```python
from build123d import *

# Parameters (mm, degrees)
SKETCH2_W                = 21
SKETCH2_H                = 21
BOSS_EXTRUDE1_DEPTH      = 300
BOSS_EXTRUDE1_DEPTH_BACK = 100
SKETCH3_W                = 16
SKETCH3_H                = 16
CUT_EXTRUDE1_DEPTH       = 800
SKETCH14_R               = 2.5
BOSS_EXTRUDE3_DEPTH      = 10
LPATTERN1_COUNT          = 3
LPATTERN1_PITCH          = 120


with BuildPart() as part:
    # Sketch2 → Boss-Extrude1 (new body, two sides)
    with BuildSketch(Plane(origin=(0, 0, 0), x_dir=(1, 0, 0), z_dir=(0, 1, 0))) as boss_extrude1_sk:
        Rectangle(SKETCH2_W, SKETCH2_H)
    extrude(amount=BOSS_EXTRUDE1_DEPTH)
    extrude(boss_extrude1_sk.sketch, amount=-BOSS_EXTRUDE1_DEPTH_BACK)

    # Sketch3 → Cut-Extrude1 (cut)
    with BuildSketch(Plane.XZ.offset(100)):
        Rectangle(SKETCH3_W, SKETCH3_H)
    extrude(amount=-CUT_EXTRUDE1_DEPTH, mode=Mode.SUBTRACT)

    # Sketch14 → Boss-Extrude3 (add)
    with BuildSketch(Plane(origin=(9.15884387, 19.641204062, 19.641204062), x_dir=(0.949705125, -0.221427386, -0.221427386), z_dir=(0.313145613, 0.671542934, 0.671542934))):
        Polygon((-12.902384486, 16.967939861), (98.008310235, -50.846644091), (103.224816692, -42.31505219), (-7.685878028, 25.499531762), align=None)
        with Locations((87.819175611, -38.756088454)):
            Circle(SKETCH14_R, mode=Mode.SUBTRACT)
    boss_extrude3 = extrude(amount=-BOSS_EXTRUDE3_DEPTH)

    # LPattern1: Boss-Extrude3 ×3
    with Locations(*[(0, i * LPATTERN1_PITCH, 0) for i in range(1, LPATTERN1_COUNT)]):
        add(boss_extrude3)


solid = part.part
```
The listing builds one solid part. Answer for the finished solid, in the listing's coordinates (mm). A direction names the side the tool comes from. Round coordinates to 2 decimals unless told otherwise and drop trailing zeros. Loops run counter-clockwise (first coordinate to the right, second up) from the corner with the lowest first, then second, coordinate; pieces in that order, holes last. Notation, with made-up numbers: (74, -30) - (78, -30) arc R27 cw to (78, -10) - close; hole circle Ø3 at (25, 35). An arc over 180 degrees is marked (long way). Use one line per item in the form item = value. Start each with the question number.
1. For a pull along X with two mould halves and no side action, classify faces 1 (the face through (-10.5, 103, 0)), 2 (the face through (103.136, -38.921, 27.039)), 3 (the face through (0, 103, -10.5)), 4 (the face through (0, 97, 8)) as pulls with the +X half, pulls with the -X half, needs draft (parallel to the pull), parting line crosses it, or undercut.
2. A tool of negligible diameter and unlimited length cuts with its end or side. For faces 5 (the face through (-2.127, 273.659, 3.545)), 6 (the face through (51.8, -1.1, 20.5)), 7 (the face through (53.6, 232.11, 11.56)), 8 (the face through (4, 153.5, 0.8)), 9 (the face through (57.98, 116.37, 12.81)), from which of +Z, -Z, +X, -X, +Y, -Y can it reach the whole face along a straight path? Write none if from no direction.
3. The part is cut by section B-B on y = 226.5. Determine the outline of the cut face in (x, z).
4. The part is cut by section A-A on y = -68.5. Determine the outline of the cut face in (x, z).
5. Given pin 1 Ø6 at (y, z) = (255.5, 20.5) entering from -X; pin 2 Ø10.5 at (y, z) = (57, -2) entering from +X; pin 3 Ø1.5 at (x, y) = (29.5, 127.5) entering from -Z; pin 4 Ø17.5 at (x, y) = (1, 75.5) entering from +Z, each flat-ended and moving along its own axis, determine where each tip first touches the part or whether it passes through.
6. The part is cut by section C-C on x = 20. Determine the outline of the cut face in (y, z).
7. Consider line 1 (X direction, y = 262, z = -1.5); line 2 (Y direction, x = 36, z = 14.5); line 3 (Y direction, x = 5.5, z = 12). Determine where each line is inside the solid, lowest interval first. Write a range as [from, to].
Geometry check:
q1.face_1 = pulls with the -X half
q1.face_2 = pulls with the +X half
q1.face_3 = needs draft
q1.face_4 = undercut
q2.face_5 = +Y
q2.face_6 = +Z, +X
q2.face_7 = -Z
q2.face_8 = none
q2.face_9 = -Z, +X
q3.outline = (-10.5, -10.5) - (10.5, -10.5) - (10.5, 10.5) - (-10.5, 10.5) - close; (53.74, 17.1) - (65.78, 11.49) - (78.67, 20.37) - (66.63, 25.98) - close; hole (-8, -8) - (8, -8) - (8, 8) - (-8, 8) - close
q4.outline = (-10.5, -10.5) - (10.5, -10.5) - (10.5, 10.5) - (-10.5, 10.5) - close; hole (-8, -8) - (8, -8) - (8, 8) - (-8, 8) - close
q5.pin_1 = through
q5.pin_2 = 10.5
q5.pin_3 = 6.58
q5.pin_4 = 10.5
q6.outline = (9.73, 9.61) - (18.01, 1.32) - (26.89, 7.34) - (18.6, 15.63) - close; (129.73, 9.61) - (138.01, 1.32) - (146.89, 7.34) - (138.6, 15.63) - close; (249.73, 9.61) - (258.01, 1.32) - (266.89, 7.34) - (258.6, 15.63) - close
q7.line_1 = [-10.5, -8], [8, 10.5]
q7.line_2 = [0.68, 12.27], [120.68, 132.27], [240.68, 252.27]
q7.line_3 = [27.98, 28.99], [147.98, 148.99], [267.98, 268.99]
